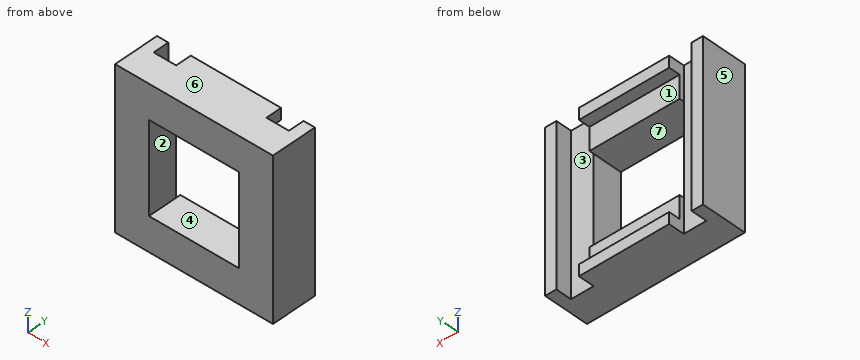
```python
from build123d import *

# Parameters (mm, degrees)
CROQUIS1_W                 = 70
CROQUIS1_H                 = 70
SALIENTE_EXTRUIR1_DEPTH    = 20
CROQUIS2_W                 = 60
CROQUIS2_H                 = 60
CORTAR_EXTRUIR1_DEPTH      = 5
CORTAR_EXTRUIR2_DEPTH      = 5
CORTAR_EXTRUIR2_DEPTH_BACK = 2
CROQUIS3_W                 = 10
CROQUIS3_H                 = 70
CROQUIS4_W                 = 40
CROQUIS4_H                 = 40
CORTAR_EXTRUIR3_DEPTH      = 52


with BuildPart() as part:
    # Croquis1 → Saliente-Extruir1 (new body)
    with BuildSketch(Plane(origin=(0, 0, 0), x_dir=(1, 0, 0), z_dir=(0, 1, 0))):
        with Locations((35, 35)):
            Rectangle(CROQUIS1_W, CROQUIS1_H)
    extrude(amount=SALIENTE_EXTRUIR1_DEPTH)

    # Croquis2 → Cortar-Extruir1 (cut)
    with BuildSketch(Plane(origin=(0, 20, 0), x_dir=(1, 0, 0), z_dir=(0, 1, 0))):
        with Locations((35, 35)):
            Rectangle(CROQUIS2_W, CROQUIS2_H)
    extrude(amount=-CORTAR_EXTRUIR1_DEPTH, mode=Mode.SUBTRACT)

    # Croquis3 → Cortar-Extruir2 (cut, two sides: drawn at the far end of the back side and taken through both)
    with BuildSketch(Plane(origin=(0, 15, 0), x_dir=(1, 0, 0), z_dir=(0, 1, 0)).offset(-CORTAR_EXTRUIR2_DEPTH_BACK)):
        with Locations((10, 35)):
            Rectangle(CROQUIS3_W, CROQUIS3_H)
        with Locations((60, 35)):
            Rectangle(CROQUIS3_W, CROQUIS3_H)
    extrude(amount=CORTAR_EXTRUIR2_DEPTH + CORTAR_EXTRUIR2_DEPTH_BACK, mode=Mode.SUBTRACT)

    # Croquis4 → Cortar-Extruir3 (cut)
    with BuildSketch(Plane(origin=(0, 15, 0), x_dir=(1, 0, 0), z_dir=(0, 1, 0))):
        with Locations((35, 35)):
            Rectangle(CROQUIS4_W, CROQUIS4_H)
    extrude(amount=-CORTAR_EXTRUIR3_DEPTH, mode=Mode.SUBTRACT)


solid = part.part
```
The model under review builds one solid part; all positions refer to its coordinate system, in mm. Face numbers are marked on the shaded views. A direction names the side the tool comes from. Coordinates: 2 decimals unless noted, no trailing zeros. Write each loop counter-clockwise with the first axis right and the second up, starting at its lowest first coordinate (ties: lowest second). Pieces come first, ordered by that corner, then holes.
1) We need section D-D on z = -14. State the section outline as (x, y) points, then the cut area to 3 significant figures.
2) To check wall thickness, follow probe 1 along X at (y, z) = (15, -45); probe 2 along Z at (x, y) = (51.5, 13); probe 3 along X at (y, z) = (12.75, -34.5). State the ranges of each line that lie inside material, in increasing order.
3) Machinability: for the marked faces 1, 2 and 3, which of the approach directions +Z, -Z, +X, -X, +Y, -Y give a long, thin tool a straight path to every point of the face, cutting with its end or side? Answer none if there is none.
4) We need section A-A on y = 4. State the section outline as (x, z) points.
5) The part is to be moulded in two halves that separate along X. For the marked faces 4, 5, 6 and 7, say which applies: pulls with the +X half, pulls with the -X half, needs draft (parallel to the pull), parting line crosses it, or undercut.
6) We need section C-C on z = -49. State the section outline as (x, y) points, then the cut area to 3 significant figures.
7) We need section B-B on x = 20.5. State the section outline as (y, z) points.
8) Clearance check with flat-ended pins moving along their axes: pin 1 Ø1.5 at (x, z) = (60, -52) entering from +Y; pin 2 Ø6 at (x, z) = (32, -12) entering from +Y. State where each tip first meets the part, or that it passes through.
Answer list:
1. outline: (0, 0) - (70, 0) - (70, 20) - (65, 20) - (65, 13) - (55, 13) - (55, 15) - (15, 15) - (15, 13) - (5, 13) - (5, 20) - (0, 20) - close
1. area: 1,060 mm2
2. probe 1: x = 0 to 5, 65 to 70
2. probe 2: z = -70 to -55, -15 to 0
2. probe 3: x = 0 to 15, 55 to 70
3. face 1: +Y
3. face 2: +Y, -Y
3. face 3: +Z, -Z, +Y
4. outline: (0, -70) - (70, -70) - (70, 0) - (0, 0) - close; hole (15, -55) - (55, -55) - (55, -15) - (15, -15) - close
5. face 4: undercut
5. face 5: pulls with the -X half
5. face 6: needs draft
5. face 7: undercut
6. outline: (0, 0) - (15, 0) - (15, 13) - (5, 13) - (5, 20) - (0, 20) - close; (55, 0) - (70, 0) - (70, 20) - (65, 20) - (65, 13) - (55, 13) - close
6. area: 460 mm2
7. outline: (0, -70) - (20, -70) - (20, -65) - (15, -65) - (15, -55) - (0, -55) - close; (0, -15) - (15, -15) - (15, -5) - (20, -5) - (20, 0) - (0, 0) - close
8. pin 1: stops at y = 13
8. pin 2: stops at y = 15
